The drawing under review shows one solid part. Ordinate dimensions are in mm from its lowest x, y, z. A direction names the side the tool comes from. Give positions to 0.01 mm unless a question says otherwise; leave off trailing zeros. Order: outer loops, then holes, each group sorted by start corner. A loop starts at its lowest first (then second) coordinate and runs counter-clockwise, first axis right, second up. Notation, with made-up numbers: (51, 34.25) -> (62, 34.25) arc R19 ccw to (62, 43.25) -> close; hole circle Ø6 at (-23, 6). An arc over 180 degrees is marked (long way). Return JSON: item names as keys, results as strings. Group by question number.
1) Add section A-A (z = 15). Give the boundary of the cut face in (x, y), then the cut area to 3 significant figures.
2) To check wall thickness, follow line 1 along X through (y, z) = (14, 5.25); line 2 along X through (y, z) = (2.15, 9); line 3 along Y through (x, z) = (1.7, 15). State the ranges of each line that lie inside material, in increasing order.
3) Add section D-D (x = 2.25). Give the boundary of the cut face in (y, z).
4) For the marked faces 4 and 5, list the 3-axis set-ups (+Z, -Z, +X, -X, +Y, -Y) from which the entire face can be reached by the end or side of a thin tool; tool diameter is ignored.
5) Add section C-C (x = 12). Give the boundary of the cut face in (y, z), then the cut area to 3 significant figures.
6) The part is to be moulded in two halves that separate along X. For the marked faces 1, 2 and 3, say which applies: released by +X, released by -X, zero draft, split by the parting line, or undercut.
7) Add section B-B (y = 16.5). Give the boundary of the cut face in (x, z).
8) Insertion check: P1, Ø10, axis at x = 14, z = 20, coming from the +Y side. The pin has a flat end and moves straight along its axis. Give the tip position at first contact, or say it passes through.
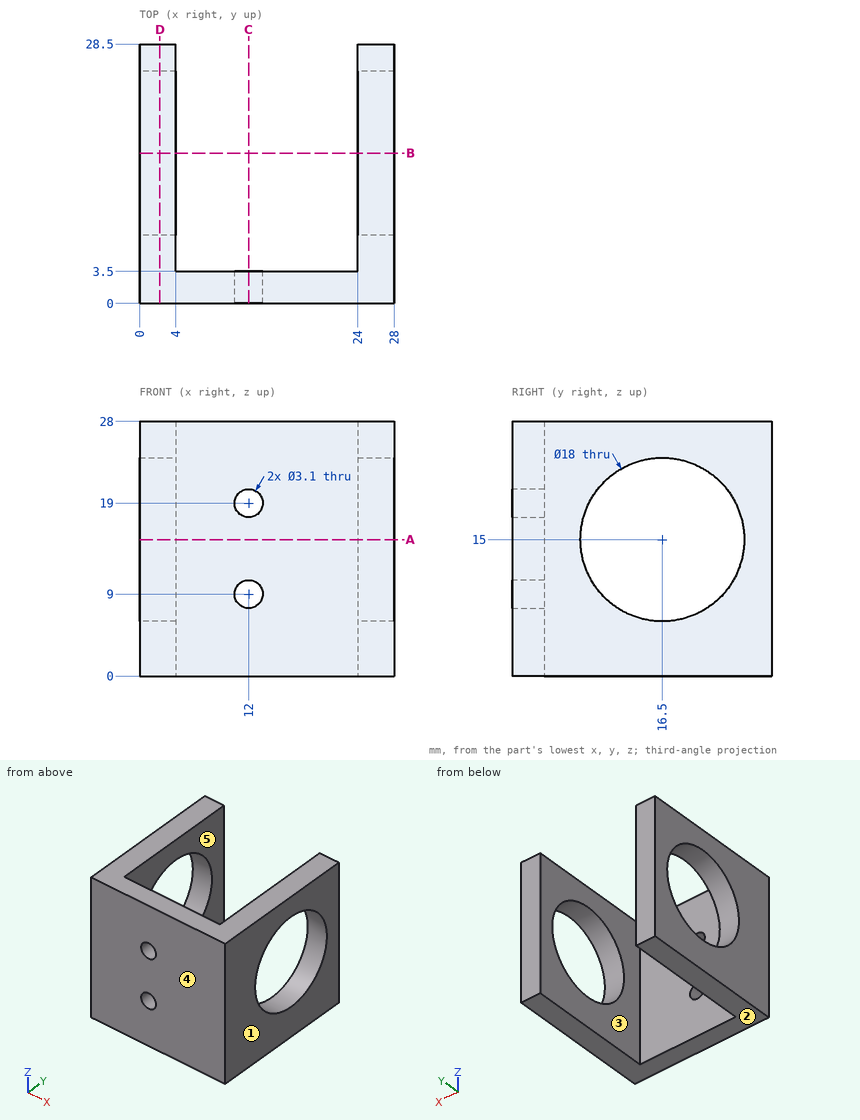
Evaluation:
{
 "1": {"outline": "(0, 0) -> (28, 0) -> (28, 7.5) -> (24, 7.5) -> (24, 3.5) -> (4, 3.5) -> (4, 7.5) -> (0, 7.5) -> close; (0, 25.5) -> (4, 25.5) -> (4, 28.5) -> (0, 28.5) -> close; (24, 25.5) -> (28, 25.5) -> (28, 28.5) -> (24, 28.5) -> close", "area": "154 mm^2"},
 "2": {"line 1": "0 to 4, 24 to 28", "line 2": "0 to 10.45, 13.55 to 28", "line 3": "0 to 7.5, 25.5 to 28.5"},
 "3": {"outline": "(0, 0) -> (28.5, 0) -> (28.5, 28) -> (0, 28) -> close; hole circle Ø18 at (16.5, 15)"},
 "4": {"face 4": "+Z, -Z, +X, -X, -Y", "face 5": "+Z, -Z, +Y"},
 "5": {"outline": "(0, 0) -> (3.5, 0) -> (3.5, 7.45) -> (0, 7.45) -> close; (0, 10.55) -> (3.5, 10.55) -> (3.5, 17.45) -> (0, 17.45) -> close; (0, 20.55) -> (3.5, 20.55) -> (3.5, 28) -> (0, 28) -> close", "area": "76.3 mm^2"},
 "6": {"face 1": "released by +X", "face 2": "zero draft", "face 3": "undercut"},
 "7": {"outline": "(0, 0) -> (4, 0) -> (4, 6) -> (0, 6) -> close; (0, 24) -> (4, 24) -> (4, 28) -> (0, 28) -> close; (24, 0) -> (28, 0) -> (28, 6) -> (24, 6) -> close; (24, 24) -> (28, 24) -> (28, 28) -> (24, 28) -> close"},
 "8": {"P1": "y = 3.5"}
}
